Verification items for the finished model (mm, model axes). Face numbers are marked on the shaded views. A direction names the side the tool comes from. Coordinates: 2 decimals unless noted, no trailing zeros. Write each loop counter-clockwise with the first axis right and the second up, starting at its lowest first coordinate (ties: lowest second). Pieces come first, ordered by that corner, then holes. Notation, with made-up numbers: M 30,19 L 39,19 A21 ccw 39,46 Z; hole C 2.5,75.25 d10. An arc over 180 degrees is marked long. One line per item, written item: value.
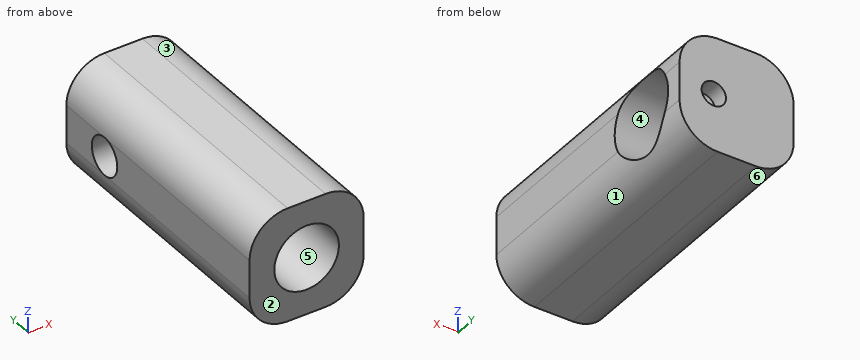
```python
from build123d import *

# Parameters (mm, degrees)
SKETCH1_W               = 15
SKETCH1_H               = 15
SKETCH1_R               = 4.25
BOSS_EXTRUDE1_DEPTH     = 20
SKETCH2_W               = 15
SKETCH2_H               = 15
BOSS_EXTRUDE2_DEPTH     = 16
SKETCH3_R               = 2.5
CUT_EXTRUDE1_DEPTH      = 40.714606885
FILLET1_R               = 5
SKETCH4_R               = 5.25
CUT_EXTRUDE2_DEPTH      = 7
CUT_EXTRUDE3_REACH      = 39.53
CUT_EXTRUDE3_END_RADIUS = 5.25
SKETCH5_R               = 1.6
CHAMFER1_SIZE           = 10
CHAMFER1_SIZE2          = 0.174550649


with BuildPart() as part:
    # Sketch1 → Boss-Extrude1 (new body)
    with BuildSketch(Plane(origin=(0, 0, 0), x_dir=(1, 0, 0), z_dir=(0, 1, 0))):
        Rectangle(SKETCH1_W, SKETCH1_H)
        with Locations(Location((0, 0, 0), (0, 0, 270))):
            Circle(SKETCH1_R, mode=Mode.SUBTRACT)
    extrude(amount=BOSS_EXTRUDE1_DEPTH)

    # Sketch2 → Boss-Extrude2 (add)
    with BuildSketch(Plane(origin=(0, 20, 0), x_dir=(1, 0, 0), z_dir=(0, 1, 0))):
        Rectangle(SKETCH2_W, SKETCH2_H)
    extrude(amount=BOSS_EXTRUDE2_DEPTH)

    # Sketch3 → Cut-Extrude1 (cut, through all)
    with BuildSketch(Plane(origin=(7.5, 0, 0), x_dir=(0, 0, -1), z_dir=(1, 0, 0))):
        with Locations((0, 28.5)):
            Circle(SKETCH3_R)
    extrude(amount=-CUT_EXTRUDE1_DEPTH, mode=Mode.SUBTRACT)

    # Fillet1
    fillet1_edges = [part.edges().sort_by_distance(p)[0] for p in [
        (-7.5, 18, -7.5),
        (7.5, 18, -7.5),
        (7.5, 18, 7.5),
        (-7.5, 18, 7.5),
    ]]
    fillet(fillet1_edges, radius=FILLET1_R - 0.0001)  # a hair under: the kernel refuses the full size

    # Sketch4 → Cut-Extrude2 (cut)
    with BuildSketch(Plane(origin=(7.5, 0, 0), x_dir=(0, 0, -1), z_dir=(1, 0, 0))):
        with Locations((0, 28.5)):
            Circle(SKETCH4_R)
    extrude(amount=-CUT_EXTRUDE2_DEPTH, mode=Mode.SUBTRACT)

    # Cut-Extrude3: up to this cylinder (the profile starts outside it)
    cut_extrude3_end = Plane(origin=(3, 28.5, 0), z_dir=(1, 0, 0)) * Cylinder(CUT_EXTRUDE3_END_RADIUS, 90.56, mode=Mode.PRIVATE)
    # Sketch5 → Cut-Extrude3 (cut, up to the surface)
    with BuildSketch(Plane(origin=(0, 36, 0), x_dir=(1, 0, 0), z_dir=(0, 1, 0)), mode=Mode.PRIVATE) as cut_extrude3_sk1:
        with Locations(Location((3, 0, 0), (0, 0, 270))):
            Circle(SKETCH5_R)
    cut_extrude3_tool1 = extrude(cut_extrude3_sk1.sketch, amount=-CUT_EXTRUDE3_REACH, mode=Mode.PRIVATE) - cut_extrude3_end
    add(cut_extrude3_tool1.solids().sort_by_distance((3, 36, 0))[0], mode=Mode.SUBTRACT)

    # Chamfer1
    chamfer1_edges = [part.edges().sort_by_distance(p)[0] for p in [
        (0, 20, -4.25),
    ]]
    chamfer1_side = [part.faces().sort_by_distance(p)[0] for p in [
        (0, 10, -4.25),
    ]]
    chamfer(chamfer1_edges, length=CHAMFER1_SIZE, length2=CHAMFER1_SIZE2, reference=chamfer1_side[0])


solid = part.part
```
Item 1: Cross-section at C-C, the plane y = 11.5. Enter the section's corners in (x, z).
The answers:
outline: M -7.5,-2.5 A5 ccw -2.5,-7.5 L 2.5,-7.5 A5 ccw 7.5,-2.5 L 7.5,2.5 A5 ccw 2.5,7.5 L -2.5,7.5 A5 ccw -7.5,2.5 Z; hole C 0,0 d8.45
Item 2: Draft check along Z on the marked faces 1, 2, 3 and 4. Enter one of: released by +Z, released by -Z, zero draft, split by the parting line, or undercut.
The answers:
face 1: released by -Z
face 2: zero draft
face 3: released by +Z
face 4: undercut
Item 3: Scan lines: line 1 (Y direction, x = -2.5, z = 0); line 2 (X direction, y = 19, z = 0.25); line 3 (X direction, y = 34.9, z = 0). Record each from-to range of solid material in increasing order.
The answers:
line 1: y = 20 to 26, 31 to 36
line 2: x = -7.5 to -4.09, 4.09 to 7.5
line 3: x = -7.5 to 1.4, 4.6 to 7.5
Item 4: Cross-section at B-B, the plane x = 5.25. Enter the section's corners in (y, z), and give its area (3 significant figures).
The answers:
outline: M 0,-6.68 L 36,-6.68 L 36,6.68 L 0,6.68 Z; hole C 28.5,0 d10.5
area: 394 mm²
Item 5: Cross-section at A-A, the plane y = 22. Enter the section's corners in (x, z), and give its area (3 significant figures).
The answers:
outline: M -7.5,-2.5 A5 ccw -2.5,-7.5 L 2.5,-7.5 A5 ccw 7.5,-2.5 L 7.5,2.5 A5 ccw 2.5,7.5 L -2.5,7.5 A5 ccw -7.5,2.5 Z
area: 204 mm²
Item 6: Access from +Z, -Z, +X, -X, +Y, -Y to the whole of each face (thin tool, end or side, straight path). Record for the marked faces 5 and 6.
The answers:
face 5: -Y
face 6: -Z, -X, +Y, -Y
Item 7: Go/stop test with a flat-tipped pin: P1, Ø2.5, axis at x = 2, z = -1, coming from the -Y side. Record where the tip stops, or that it passes through.
The answers:
P1: stops at y = 20
Item 8: Cross-section at D-D, the plane z = 0. Give the number of separate pieces and of enclosed holes in the cut face, and give its area (3 significant figures).
The answers:
separate pieces: 3
enclosed holes: 0
area: 251 mm²
